Build history of the part. All positions in model axes, mm. A direction names the side the tool comes from. Coordinates: 2 decimals unless noted, no trailing zeros. Loops run counter-clockwise (first coordinate to the right, second up) from the corner with the lowest first, then second, coordinate; pieces in that order, holes last.
(1) Two-plate mould, pull along X, no slides. Class faces 1 (the face through (0, -2.93, -3)), 2 (the face through (5.73, -1.96, 2.36)), 3 (the face through (1.46, 0, 2)): pulls with the +X half, pulls with the -X half, needs draft (parallel to the pull), parting line crosses it, or undercut.
(2) Tool access for faces 4 (the face through (-0.765, 0, -4)), 5 (the face through (2.765, 0, -6)), 6 (the face through (-2.04, -1.92, 2.36)): list every direction of +Z, -Z, +X, -X, +Y, -Y with a clear straight run to the whole face (end or side of a thin tool).
(3) Flat gauge pins, fed straight in: P1, Ø0.8, axis at x = 3.5, z = 1.5, coming from the +Y side; P2, Ø0.8, axis at y = 0, z = -6, coming from the -X side (3 decimals); P3, Ø1.2, axis at x = -4, z = 2.5, coming from the -Y side; P4, Ø1, axis at x = 0.5, z = 1.5, coming from the -Y side. Where does each tip first touch, or does it go through?
(4) Slice it at D-D (z = -3). Give the cut face in (x, y) (3 decimals), and give its area (3 significant figures).
(5) Wall check: L1, parallel to X at y = 0, z = 3.6; L2, parallel to Y at x = 3.9, z = 3.7; L3, parallel to Z at x = -3.5, y = -0.5. Give the ranges that are in metal, low to high.
(6) Slice it at C-C (y = -1.75). Give the cut face in (x, z) (3 decimals), and give its area (3 significant figures).
(7) Slice it at A-A (z = 2). Give the cut face in (x, y), and give its area (3 significant figures).
(8) Slice it at B-B (x = 0.5). Give the cut face in (y, z), and give its area (3 significant figures).
from build123d import *

# Parameters (mm, degrees)
F0_W     = 14.49
F0_H     = 7.86
F1_DEPTH = 2.16
F2_W     = 1.53
F2_H     = 7.86
F3_DEPTH = 7.02
F5_DEPTH = 8.011
F4_R     = 1.25
F6_DEPTH = 2
F9_DEPTH = 4.79


with BuildPart() as f1:
    # F0 (on Top) → F1 (new body)
    with BuildSketch(Plane.XY):
        Rectangle(F0_W, F0_H)
    extrude(amount=-F1_DEPTH)

    # F2 (on face) → F3 (join)
    with BuildSketch(Plane(origin=(0, 0, -2.16), x_dir=(1, 0, 0), z_dir=(0, 0, -1))):
        Rectangle(F2_W, F2_H)
    extrude(amount=F3_DEPTH)

    # F4 (on face) → F5 (cut, through all)
    with BuildSketch(Plane.YZ.offset(0.765)):
        with BuildLine():
            Line((-3.93, -9.18), (0, -9.18))
            ThreePointArc((0, -9.18), (-3.090612, -7.333797), (-2.93, -3.737333))
            Line((-2.93, -3.737333), (-2.93, -2.16))
            Line((-2.93, -2.16), (-3.93, -2.16))
            Line((-3.93, -2.16), (-3.93, -9.18))
        make_face()
        with BuildLine():
            ThreePointArc((2.93, -3.737333), (3.361874, -4.66109), (3.51, -5.67))
            ThreePointArc((3.51, -5.67), (2.481945, -8.151945), (0, -9.18))
            Line((0, -9.18), (3.93, -9.18))
            Line((3.93, -9.18), (3.93, -2.16))
            Line((3.93, -2.16), (2.93, -2.16))
            Line((2.93, -2.16), (2.93, -3.737333))
        make_face()
    extrude(amount=-F5_DEPTH, mode=Mode.SUBTRACT)

    # F4 (on face) → F6 (join)
    with BuildSketch(Plane.YZ.offset(0.765)):
        with Locations((0, -5.67)):
            Circle(F4_R)
    extrude(amount=F6_DEPTH)

    # F7: F1 across plane


with BuildPart() as f1_1:
    add(f1.part)
    add(f1.part.mirror(Plane.YZ))

    # F8 (on face) → F9 (join)
    with BuildSketch(Plane.XY):
        Polygon((4.95944, 2.44), (2.45944, 2.44), (1.46, 1.238976), (1.46, -1.421024), (2.644494, -2.44), (5.144494, -2.44), (6.34, -1.458122), (6.34, 1.741878), align=None)
        with BuildLine():
            ThreePointArc((5.34, 1.387948), (5.754724, 0.748331), (5.9, 0))
            ThreePointArc((5.9, 0), (5.754724, -0.748331), (5.34, -1.387948))
            ThreePointArc((5.34, -1.387948), (1.9, 0), (5.34, 1.387948))
        make_face(mode=Mode.SUBTRACT)
        with BuildLine():
            ThreePointArc((5.34, -1.387948), (5.754724, -0.748331), (5.9, 0))
            ThreePointArc((5.9, 0), (5.754724, 0.748331), (5.34, 1.387948))
            Line((5.34, 1.387948), (5.34, -1.387948))
        make_face()
    extrude(amount=F9_DEPTH)

    # F10: F1 across plane


with BuildPart() as f1_2:
    add(f1_1.part)
    add(f1_1.part.mirror(Plane.YZ))


solid = f1_2.part
Response values:
1. face 1: needs draft
1. face 2: pulls with the +X half
1. face 3: undercut
2. face 4: -X
2. face 5: -Z, +X, +Y, -Y
2. face 6: +Z, -Y
3. P1: stops at y = 2.44
3. P2: stops at x = -2.765
3. P3: stops at y = -2.44
3. P4: passes through
4. outline: (-0.765, -2.93) - (0.765, -2.93) - (0.765, 2.93) - (-0.765, 2.93) - close
4. area: 8.97 mm2
5. L1: x = -6.34 to -5.34, -1.9 to -1.46, 1.46 to 1.9, 5.34 to 6.34
5. L2: y = -2.44 to -2, 2 to 2.44
5. L3: z = -2.16 to 0
6. outline: (-7.245, -2.16) - (-0.765, -2.16) - (-0.765, -8.713) - (0.765, -8.713) - (0.765, -2.16) - (7.245, -2.16) - (7.245, 0) - (5.985, 0) - (5.985, 4.79) - (4.868, 4.79) - (4.868, 0) - (2.932, 0) - (2.932, 4.79) - (1.842, 4.79) - (1.842, 0) - (-1.842, 0) - (-1.842, 4.79) - (-2.932, 4.79) - (-2.932, 0) - (-4.868, 0) - (-4.868, 4.79) - (-5.985, 4.79) - (-5.985, 0) - (-7.245, 0) - close
6. area: 62.5 mm2
7. outline: (-6.34, -1.46) - (-5.14, -2.44) - (-2.64, -2.44) - (-1.46, -1.42) - (-1.46, 1.24) - (-2.46, 2.44) - (-4.96, 2.44) - (-6.34, 1.74) - close; (1.46, -1.42) - (2.64, -2.44) - (5.14, -2.44) - (6.34, -1.46) - (6.34, 1.74) - (4.96, 2.44) - (2.46, 2.44) - (1.46, 1.24) - close; hole (-5.34, -1.39) arc R2 ccw (long way) to (-5.34, 1.39) - close; hole (5.34, -1.39) - (5.34, 1.39) arc R2 ccw (long way) to start
7. area: 20.1 mm2
8. outline: (-3.93, -2.16) - (-2.93, -2.16) - (-2.93, -3.74) arc R3.51 ccw to (0, -9.18) arc R3.51 ccw to (3.51, -5.67) arc R3.51 ccw to (2.93, -3.74) - (2.93, -2.16) - (3.93, -2.16) - (3.93, 0) - (-3.93, 0) - close
8. area: 58.4 mm2
